from build123d import *

# Parameters (mm, degrees)
SKETCH1_R           = 11
BOSS_EXTRUDE1_DEPTH = 5
FILLET1_R           = 1
FILLET2_R           = 1
FILLET3_R           = 1
FILLET4_R           = 1
FILLET5_R           = 1
FILLET6_R           = 1
FILLET7_R           = 1
FILLET8_R           = 1


with BuildPart() as part:
    # Sketch1 → Boss-Extrude1 (new body)
    with BuildSketch(Plane(origin=(0, 0, 0), x_dir=(1, 0, 0), z_dir=(0, 1, 0))):
        Polygon((8.83016903, -15), (17.405465572, 0.1471507), (8.575296542, 15.1471507), (-8.83016903, 15), (-17.405465572, -0.1471507), (-8.575296542, -15.1471507), align=None)
        with Locations(Location((0, 0, 0), (0, 0, 270))):
            Circle(SKETCH1_R, mode=Mode.SUBTRACT)
    extrude(amount=BOSS_EXTRUDE1_DEPTH)

    # Fillet1
    fillet1_edges = [part.edges().sort_by_distance(p)[0] for p in [
        (-12.990381057, 0, 7.6471507),
        (-13.117817301, 0, -7.42642465),
        (-0.127436244, 0, -15.07357535),
        (12.990381057, 0, -7.6471507),
        (13.117817301, 0, 7.42642465),
        (0.127436244, 0, 15.07357535),
    ]]
    fillet(fillet1_edges, radius=FILLET1_R)

    # Fillet2
    fillet2_edges = [part.edges().sort_by_distance(p)[0] for p in [
        (12.990381057, 5, -7.6471507),
        (-0.127436244, 5, -15.07357535),
        (-13.117817301, 5, -7.42642465),
        (-12.990381057, 5, 7.6471507),
        (0.127436244, 5, 15.07357535),
        (13.117817301, 5, 7.42642465),
    ]]
    fillet(fillet2_edges, radius=FILLET2_R)

    # Fillet3
    # the kernel refuses this fillet: 1 mm, written as the material it takes off along each edge
    with BuildSketch(Plane(origin=(8.244385414, 1, 14.004916643), x_dir=(0.870221445448491, 0, 0.4926607716081514), z_dir=(0, -1, 0))) as fillet3_piece_1_section:
        Polygon((0, 0), (FILLET3_R, 0), (FILLET3_R, FILLET3_R * 0.57735026919), (FILLET3_R * 0.5, FILLET3_R * 0.866025403784), align=None)
    fillet3_piece_1 = extrude(amount=FILLET3_R, mode=Mode.PRIVATE)
    fillet3_piece_1 = fillet3_piece_1 - Plane(origin=(8.244385414, 1, 14.004916643), x_dir=(-0.5073034928723316, 0, -0.8617674663849478), z_dir=(0, -1, 0)) * Sphere(FILLET3_R, mode=Mode.PRIVATE)
    add(fillet3_piece_1, mode=Mode.SUBTRACT)
    with BuildSketch(Plane(origin=(8.244385414, 4, 14.004916643), x_dir=(0.870221445448491, 0, 0.4926607716081514), z_dir=(0, 1, 0))) as fillet3_piece_2_section:
        Polygon((0, 0), (FILLET3_R, 0), (FILLET3_R, -FILLET3_R * 0.57735026919), (FILLET3_R * 0.5, -FILLET3_R * 0.866025403784), align=None)
    fillet3_piece_2 = extrude(amount=FILLET3_R, mode=Mode.PRIVATE)
    fillet3_piece_2 = fillet3_piece_2 - Plane(origin=(8.244385414, 4, 14.004916643), x_dir=(-0.5073034928723316, 0, -0.8617674663849478), z_dir=(0, 1, 0)) * Sphere(FILLET3_R, mode=Mode.PRIVATE)
    add(fillet3_piece_2, mode=Mode.SUBTRACT)
    with BuildSketch(Plane(origin=(8.83016903, 1, 15), x_dir=(0.4926607716081517, 0, -0.8702214454484907), z_dir=(0, 1, 0))) as fillet3_piece_3:
        with BuildLine():
            CenterArc((FILLET3_R * 0.57735026919, FILLET3_R), FILLET3_R, 210, 60)
            Line((-FILLET3_R * 0.288675134595, FILLET3_R * 0.5), (0, 0))
            Line((0, 0), (FILLET3_R * 0.57735026919, 0))
        make_face()
    extrude(amount=3, mode=Mode.SUBTRACT)

    # Fillet4
    # the kernel refuses this fillet: 1 mm, written as the material it takes off along each edge
    with BuildSketch(Plane(origin=(-8.006420883, 1, 14.142305528), x_dir=(0.008453979063543083, 0, 0.999964264480483), z_dir=(0, -1, 0))) as fillet4_piece_1_section:
        Polygon((0, 0), (FILLET4_R, 0), (FILLET4_R, FILLET4_R * 0.57735026919), (FILLET4_R * 0.5, FILLET4_R * 0.866025403784), align=None)
    fillet4_piece_1 = extrude(amount=FILLET4_R, mode=Mode.PRIVATE)
    fillet4_piece_1 = fillet4_piece_1 - Plane(origin=(-8.006420883, 1, 14.142305528), x_dir=(0.49266077160815147, 0, -0.870221445448491), z_dir=(0, -1, 0)) * Sphere(FILLET4_R, mode=Mode.PRIVATE)
    add(fillet4_piece_1, mode=Mode.SUBTRACT)
    with BuildSketch(Plane(origin=(-8.006420883, 4, 14.142305528), x_dir=(0.008453979063543083, 0, 0.999964264480483), z_dir=(0, 1, 0))) as fillet4_piece_2_section:
        Polygon((0, 0), (FILLET4_R, 0), (FILLET4_R, -FILLET4_R * 0.57735026919), (FILLET4_R * 0.5, -FILLET4_R * 0.866025403784), align=None)
    fillet4_piece_2 = extrude(amount=FILLET4_R, mode=Mode.PRIVATE)
    fillet4_piece_2 = fillet4_piece_2 - Plane(origin=(-8.006420883, 4, 14.142305528), x_dir=(0.49266077160815147, 0, -0.870221445448491), z_dir=(0, 1, 0)) * Sphere(FILLET4_R, mode=Mode.PRIVATE)
    add(fillet4_piece_2, mode=Mode.SUBTRACT)
    with BuildSketch(Plane(origin=(-8.575296542, 1, 15.1471507), x_dir=(0.9999642644804829, 0, -0.008453979063542578), z_dir=(0, 1, 0))) as fillet4_piece_3:
        with BuildLine():
            CenterArc((FILLET4_R * 0.57735026919, FILLET4_R), FILLET4_R, 210, 60)
            Line((-FILLET4_R * 0.288675134595, FILLET4_R * 0.5), (0, 0))
            Line((0, 0), (FILLET4_R * 0.57735026919, 0))
        make_face()
    extrude(amount=3, mode=Mode.SUBTRACT)

    # Fillet5
    # the kernel refuses this fillet: 1 mm, written as the material it takes off along each edge
    with BuildSketch(Plane(origin=(-16.250806297, 1, 0.137388886), x_dir=(-0.870221445448491, 0, -0.49266077160815136), z_dir=(0, -1, 0))) as fillet5_piece_1_section:
        Polygon((0, 0), (FILLET5_R, 0), (FILLET5_R, -FILLET5_R * 0.57735026919), (FILLET5_R * 0.5, -FILLET5_R * 0.866025403784), align=None)
    fillet5_piece_1 = extrude(amount=FILLET5_R, mode=Mode.PRIVATE)
    fillet5_piece_1 = fillet5_piece_1 - Plane(origin=(-16.250806297, 1, 0.137388886), x_dir=(0.9999642644804829, 0, -0.008453979063543034), z_dir=(0, -1, 0)) * Sphere(FILLET5_R, mode=Mode.PRIVATE)
    add(fillet5_piece_1, mode=Mode.SUBTRACT)
    with BuildSketch(Plane(origin=(-16.250806297, 4, 0.137388886), x_dir=(-0.870221445448491, 0, -0.49266077160815136), z_dir=(0, 1, 0))) as fillet5_piece_2_section:
        Polygon((0, 0), (FILLET5_R, 0), (FILLET5_R, FILLET5_R * 0.57735026919), (FILLET5_R * 0.5, FILLET5_R * 0.866025403784), align=None)
    fillet5_piece_2 = extrude(amount=FILLET5_R, mode=Mode.PRIVATE)
    fillet5_piece_2 = fillet5_piece_2 - Plane(origin=(-16.250806297, 4, 0.137388886), x_dir=(0.9999642644804829, 0, -0.008453979063543034), z_dir=(0, 1, 0)) * Sphere(FILLET5_R, mode=Mode.PRIVATE)
    add(fillet5_piece_2, mode=Mode.SUBTRACT)
    with BuildSketch(Plane(origin=(-17.405465572, 1, 0.1471507), x_dir=(0.4926607716081488, 0, -0.8702214454484924), z_dir=(0, 1, 0))) as fillet5_piece_3:
        with BuildLine():
            CenterArc((FILLET5_R * 0.57735026919, -FILLET5_R), FILLET5_R, 90, 60)
            Line((-FILLET5_R * 0.288675134595, -FILLET5_R * 0.5), (0, 0))
            Line((0, 0), (FILLET5_R * 0.57735026919, 0))
        make_face()
    extrude(amount=3, mode=Mode.SUBTRACT)

    # Fillet6
    # the kernel refuses this fillet: 1 mm, written as the material it takes off along each edge
    with BuildSketch(Plane(origin=(-8.244385414, 1, -14.004916643), x_dir=(-0.008453979063543077, 0, -0.9999642644804829), z_dir=(0, -1, 0))) as fillet6_piece_1_section:
        Polygon((0, 0), (FILLET6_R, 0), (FILLET6_R, -FILLET6_R * 0.57735026919), (FILLET6_R * 0.5, -FILLET6_R * 0.866025403784), align=None)
    fillet6_piece_1 = extrude(amount=FILLET6_R, mode=Mode.PRIVATE)
    fillet6_piece_1 = fillet6_piece_1 - Plane(origin=(-8.244385414, 1, -14.004916643), x_dir=(0.5073034928723316, 0, 0.8617674663849478), z_dir=(0, -1, 0)) * Sphere(FILLET6_R, mode=Mode.PRIVATE)
    add(fillet6_piece_1, mode=Mode.SUBTRACT)
    with BuildSketch(Plane(origin=(-8.244385414, 4, -14.004916643), x_dir=(-0.008453979063543077, 0, -0.9999642644804829), z_dir=(0, 1, 0))) as fillet6_piece_2_section:
        Polygon((0, 0), (FILLET6_R, 0), (FILLET6_R, FILLET6_R * 0.57735026919), (FILLET6_R * 0.5, FILLET6_R * 0.866025403784), align=None)
    fillet6_piece_2 = extrude(amount=FILLET6_R, mode=Mode.PRIVATE)
    fillet6_piece_2 = fillet6_piece_2 - Plane(origin=(-8.244385414, 4, -14.004916643), x_dir=(0.5073034928723316, 0, 0.8617674663849478), z_dir=(0, 1, 0)) * Sphere(FILLET6_R, mode=Mode.PRIVATE)
    add(fillet6_piece_2, mode=Mode.SUBTRACT)
    with BuildSketch(Plane(origin=(-8.83016903, 1, -15), x_dir=(0.9999642644804829, 0, -0.008453979063542578), z_dir=(0, 1, 0))) as fillet6_piece_3:
        with BuildLine():
            CenterArc((FILLET6_R * 0.57735026919, -FILLET6_R), FILLET6_R, 90, 60)
            Line((-FILLET6_R * 0.288675134595, -FILLET6_R * 0.5), (0, 0))
            Line((0, 0), (FILLET6_R * 0.57735026919, 0))
        make_face()
    extrude(amount=3, mode=Mode.SUBTRACT)

    # Fillet7
    # the kernel refuses this fillet: 1 mm, written as the material it takes off along each edge
    with BuildSketch(Plane(origin=(8.006420883, 1, -14.142305528), x_dir=(0.8617674663849478, 0, -0.5073034928723317), z_dir=(0, -1, 0))) as fillet7_piece_1_section:
        Polygon((0, 0), (FILLET7_R, 0), (FILLET7_R, -FILLET7_R * 0.57735026919), (FILLET7_R * 0.5, -FILLET7_R * 0.866025403784), align=None)
    fillet7_piece_1 = extrude(amount=FILLET7_R, mode=Mode.PRIVATE)
    fillet7_piece_1 = fillet7_piece_1 - Plane(origin=(8.006420883, 1, -14.142305528), x_dir=(-0.4926607716081513, 0, 0.870221445448491), z_dir=(0, -1, 0)) * Sphere(FILLET7_R, mode=Mode.PRIVATE)
    add(fillet7_piece_1, mode=Mode.SUBTRACT)
    with BuildSketch(Plane(origin=(8.006420883, 4, -14.142305528), x_dir=(0.8617674663849478, 0, -0.5073034928723317), z_dir=(0, 1, 0))) as fillet7_piece_2_section:
        Polygon((0, 0), (FILLET7_R, 0), (FILLET7_R, FILLET7_R * 0.57735026919), (FILLET7_R * 0.5, FILLET7_R * 0.866025403784), align=None)
    fillet7_piece_2 = extrude(amount=FILLET7_R, mode=Mode.PRIVATE)
    fillet7_piece_2 = fillet7_piece_2 - Plane(origin=(8.006420883, 4, -14.142305528), x_dir=(-0.4926607716081513, 0, 0.870221445448491), z_dir=(0, 1, 0)) * Sphere(FILLET7_R, mode=Mode.PRIVATE)
    add(fillet7_piece_2, mode=Mode.SUBTRACT)
    with BuildSketch(Plane(origin=(8.575296542, 1, -15.1471507), x_dir=(0.507303492872331, 0, 0.8617674663849483), z_dir=(0, 1, 0))) as fillet7_piece_3:
        with BuildLine():
            CenterArc((FILLET7_R * 0.57735026919, -FILLET7_R), FILLET7_R, 90, 60)
            Line((-FILLET7_R * 0.288675134595, -FILLET7_R * 0.5), (0, 0))
            Line((0, 0), (FILLET7_R * 0.57735026919, 0))
        make_face()
    extrude(amount=3, mode=Mode.SUBTRACT)

    # Fillet8
    # the kernel refuses this fillet: 1 mm, written as the material it takes off along each edge
    with BuildSketch(Plane(origin=(16.250806297, 1, -0.137388886), x_dir=(0.870221445448491, 0, 0.4926607716081514), z_dir=(0, -1, 0))) as fillet8_piece_1_section:
        Polygon((0, 0), (FILLET8_R, 0), (FILLET8_R, -FILLET8_R * 0.57735026919), (FILLET8_R * 0.5, -FILLET8_R * 0.866025403784), align=None)
    fillet8_piece_1 = extrude(amount=FILLET8_R, mode=Mode.PRIVATE)
    fillet8_piece_1 = fillet8_piece_1 - Plane(origin=(16.250806297, 1, -0.137388886), x_dir=(-0.9999642644804829, 0, 0.00845397906354313), z_dir=(0, -1, 0)) * Sphere(FILLET8_R, mode=Mode.PRIVATE)
    add(fillet8_piece_1, mode=Mode.SUBTRACT)
    with BuildSketch(Plane(origin=(16.250806297, 4, -0.137388886), x_dir=(0.870221445448491, 0, 0.4926607716081514), z_dir=(0, 1, 0))) as fillet8_piece_2_section:
        Polygon((0, 0), (FILLET8_R, 0), (FILLET8_R, FILLET8_R * 0.57735026919), (FILLET8_R * 0.5, FILLET8_R * 0.866025403784), align=None)
    fillet8_piece_2 = extrude(amount=FILLET8_R, mode=Mode.PRIVATE)
    fillet8_piece_2 = fillet8_piece_2 - Plane(origin=(16.250806297, 4, -0.137388886), x_dir=(-0.9999642644804829, 0, 0.00845397906354313), z_dir=(0, 1, 0)) * Sphere(FILLET8_R, mode=Mode.PRIVATE)
    add(fillet8_piece_2, mode=Mode.SUBTRACT)
    with BuildSketch(Plane(origin=(17.405465572, 1, -0.1471507), x_dir=(-0.4926607716081509, 0, 0.8702214454484912), z_dir=(0, 1, 0))) as fillet8_piece_3:
        with BuildLine():
            CenterArc((FILLET8_R * 0.57735026919, -FILLET8_R), FILLET8_R, 90, 60)
            Line((-FILLET8_R * 0.288675134595, -FILLET8_R * 0.5), (0, 0))
            Line((0, 0), (FILLET8_R * 0.57735026919, 0))
        make_face()
    extrude(amount=3, mode=Mode.SUBTRACT)


solid = part.part
Read the model definition and answer for the solid it produces. Units are mm, in the model's axes. A direction names the side the tool comes from. Round coordinates to 2 decimals unless told otherwise and drop trailing zeros. Write each loop counter-clockwise with the first axis right and the second up, starting at its lowest first coordinate (ties: lowest second). Pieces come first, ordered by that corner, then holes.
1. Straight lines are drawn through the part: L1, parallel to X at y = 2.4, z = 0; L2, parallel to Z at x = -6, y = 1.05; L3, parallel to Y at x = 10, z = 11. For each, find the intervals that lie inside material, in ascending order.
2. Determine the mould class of faces 1 (the face through (11, 0, -3)), 2 (the face through (13.048, 2.479, -7.549)), 3 (the face through (-13.048, 2.479, 7.549)) for opening direction X: pulls with the +X half, pulls with the -X half, needs draft (parallel to the pull), parting line crosses it, or undercut.
3. Given pin 1 Ø3 at (x, y) = (-1.5, 2.5) entering from -Z; pin 2 Ø1 at (x, y) = (-0.5, 3) entering from +Z; pin 3 Ø2 at (x, y) = (-5, 4) entering from -Z, each flat-ended and moving along its own axis, determine where each tip first touches the part or whether it passes through.
4. Which of the six approach directions +Z, -Z, +X, -X, +Y, -Y give full straight-line access (tool end or side, diameter ignored) to faces 4 (the face through (0.239, 0.301, 14.787)), 5 (the face through (-0.239, 4.715, -14.772)), 6 (the face through (-8.745, 2.479, -14.87)), 7 (the face through (-0.239, 0.301, -14.787))?
5. The part is cut by section A-A, the plane y = 1.45. Determine the outline of the cut face in (x, z).
Values:
1. L1: x = -17.24 to -11, 11 to 17.24
1. L2: z = -15.02 to -9.22, 9.22 to 15.13
1. L3: y = 0 to 5
2. face 1: needs draft
2. face 2: pulls with the +X half
2. face 3: pulls with the -X half
3. pin 1: stops at z = -15.07
3. pin 2: stops at z = 15.08
3. pin 3: stops at z = -15.04
4. face 4: +Z, +X, -Y
4. face 5: -Z, -X, +Y
4. face 6: -Z, -X, +Y, -Y
4. face 7: -Z, -X, -Y
5. outline: (-17.12, -0.36) - (-9.11, -14.5) arc R1 ccw to (-8.25, -15) - (8, -15.14) arc R1 ccw to (8.87, -14.65) - (17.11, -0.64) arc R1 ccw to (17.12, 0.36) - (9.11, 14.5) arc R1 ccw to (8.25, 15) - (-8, 15.14) arc R1 ccw to (-8.87, 14.65) - (-17.11, 0.64) arc R1 ccw to start; hole circle Ø22 at (0, 0)
